Check sheet for the modelled part. Datum: model origin and axes. Units: mm. Face numbers are marked on the shaded views. A direction names the side the tool comes from. Give positions to 0.01 mm unless a question says otherwise; leave off trailing zeros. Loops run counter-clockwise (first coordinate to the right, second up) from the corner with the lowest first, then second, coordinate; pieces in that order, holes last.
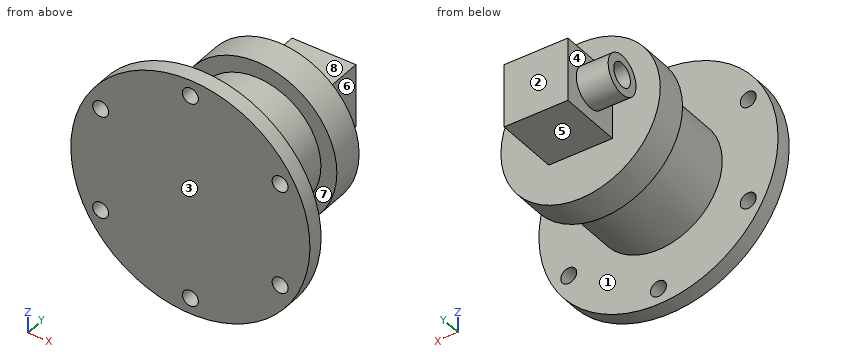
```python
from build123d import *

# Parameters (mm, degrees)
SKETCH1_R           = 75
BOSS_EXTRUDE1_DEPTH = 10
SKETCH2_R           = 5
CUT_EXTRUDE1_DEPTH  = 10
SKETCH3_R           = 40
BOSS_EXTRUDE2_DEPTH = 50
SKETCH4_R           = 50
BOSS_EXTRUDE3_DEPTH = 20
SKETCH5_W           = 40
SKETCH5_H           = 40
BOSS_EXTRUDE4_DEPTH = 40
SKETCH6_R           = 12.5
BOSS_EXTRUDE5_DEPTH = 20
SKETCH9_R           = 7.5
CUT_EXTRUDE2_DEPTH  = 15


with BuildPart() as part:
    # Sketch1 → Boss-Extrude1 (new body)
    with BuildSketch(Plane(origin=(0, 0, 0), x_dir=(1, 0, 0), z_dir=(0, 1, 0))):
        with Locations(Location((0, 0, 0), (0, 0, 270))):
            Circle(SKETCH1_R)
    extrude(amount=BOSS_EXTRUDE1_DEPTH)

    # Sketch2 → Cut-Extrude1 (cut)
    with BuildSketch(Plane(origin=(0, 10, 0), x_dir=(1, 0, 0), z_dir=(0, 1, 0))):
        with Locations(Location((0, 65, 0), (0, 0, 270))):
            Circle(SKETCH2_R)
        with Locations(Location((56.291651246, 32.5, 0), (0, 0, 270))):
            Circle(SKETCH2_R)
        with Locations(Location((56.291651246, -32.5, 0), (0, 0, 270))):
            Circle(SKETCH2_R)
        with Locations(Location((0, -65, 0), (0, 0, 270))):
            Circle(SKETCH2_R)
        with Locations(Location((-56.291651246, -32.5, 0), (0, 0, 270))):
            Circle(SKETCH2_R)
        with Locations(Location((-56.291651246, 32.5, 0), (0, 0, 270))):
            Circle(SKETCH2_R)
    extrude(amount=-CUT_EXTRUDE1_DEPTH, mode=Mode.SUBTRACT)

    # Sketch3 → Boss-Extrude2 (add)
    with BuildSketch(Plane(origin=(0, 10, 0), x_dir=(1, 0, 0), z_dir=(0, 1, 0))):
        with Locations(Location((0, 0, 0), (0, 0, 270))):
            Circle(SKETCH3_R)
    extrude(amount=BOSS_EXTRUDE2_DEPTH)

    # Sketch4 → Boss-Extrude3 (add)
    with BuildSketch(Plane(origin=(0, 60, 0), x_dir=(1, 0, 0), z_dir=(0, 1, 0))):
        with Locations(Location((0, 0, 0), (0, 0, 270))):
            Circle(SKETCH4_R)
    extrude(amount=BOSS_EXTRUDE3_DEPTH)

    # Sketch5 → Boss-Extrude4 (add)
    with BuildSketch(Plane(origin=(0, 80, 0), x_dir=(1, 0, 0), z_dir=(0, 1, 0))):
        Rectangle(SKETCH5_W, SKETCH5_H)
    extrude(amount=BOSS_EXTRUDE4_DEPTH)

    # Sketch6 → Boss-Extrude5 (add)
    with BuildSketch(Plane.ZY.offset(20)):
        with Locations(Location((0, 100, 0), (0, 0, 180))):
            Circle(SKETCH6_R)
    extrude(amount=BOSS_EXTRUDE5_DEPTH)

    # Sketch9 → Cut-Extrude2 (cut)
    with BuildSketch(Plane.ZY.offset(40)):
        with Locations((0, 100)):
            Circle(SKETCH9_R)
    extrude(amount=-CUT_EXTRUDE2_DEPTH, mode=Mode.SUBTRACT)


solid = part.part
```
(1) Section check A-A on z = 32.5. Record the boundary of the cut face in (x, y), plus the area to 3 significant figures.
(2) Section check B-B on z = 65. Record the boundary of the cut face in (x, y).
(3) Access from +Z, -Z, +X, -X, +Y, -Y to the whole of each face (thin tool, end or side, straight path). Record for the marked faces 4, 5, 6, 7 and 8.
(4) Release check for a two-part mould opening along Y. For the marked faces 1, 2 and 3 record: pulls with the +Y half, pulls with the -Y half, needs draft (parallel to the pull), parting line crosses it, or undercut.
(5) Gauge pin test, flat ends, axial feed: pin 1 Ø19.5 at (y, z) = (100, 0) entering from -X; pin 2 Ø6 at (x, y) = (31, 84) entering from -Z; pin 3 Ø5 at (x, z) = (26, 44) entering from +Y; pin 4 Ø8 at (x, y) = (26, 65) entering from +Z. Record the tip position at first contact, or that the pin passes through.
(6) Section check C-C on y = 100. Record the boundary of the cut face in (x, z), plus the area to 4 significant figures.
(7) Material ranges on line 1 (Y direction, x = -33, z = -28.5); line 2 (X direction, y = 3.75, z = 32.5); line 3 (X direction, y = 3, z = -32), recorded low to high.
(8) Section check D-D on x = 59. Record the boundary of the cut face in (y, z).
Computed values:
1. outline: (-67.59, 0) - (-61.29, 0) - (-61.29, 10) - (-67.59, 10) - close; (-51.29, 0) - (51.29, 0) - (51.29, 10) - (23.32, 10) - (23.32, 60) - (38, 60) - (38, 80) - (-38, 80) - (-38, 60) - (-23.32, 60) - (-23.32, 10) - (-51.29, 10) - close; (61.29, 0) - (67.59, 0) - (67.59, 10) - (61.29, 10) - close
1. area: 5,000 mm2
2. outline: (-37.42, 0) - (-5, 0) - (-5, 10) - (-37.42, 10) - close; (5, 0) - (37.42, 0) - (37.42, 10) - (5, 10) - close
3. face 4: -X
3. face 5: -Z, +X, -X, +Y
3. face 6: +Z, -Z, +X, +Y
3. face 7: none
3. face 8: +Z, +X, -X, +Y
4. face 1: undercut
4. face 2: pulls with the +Y half
4. face 3: pulls with the -Y half
5. pin 1: stops at x = -40
5. pin 2: passes through
5. pin 3: stops at y = 80
5. pin 4: stops at z = 44.9
6. outline: (-40, -12.5) - (-20, -12.5) - (-20, -20) - (20, -20) - (20, 20) - (-20, 20) - (-20, 12.5) - (-40, 12.5) - (-40, 7.5) - (-25, 7.5) - (-25, -7.5) - (-40, -7.5) - close
6. area: 1,875 mm2
7. line 1: y = 0 to 10, 60 to 80
7. line 2: x = -67.59 to -61.29, -51.29 to 51.29, 61.29 to 67.59
7. line 3: x = -67.83 to -61.27, -51.32 to 51.32, 61.27 to 67.83
8. outline: (0, -46.3) - (10, -46.3) - (10, -36.7) - (0, -36.7) - close; (0, -28.3) - (10, -28.3) - (10, 28.3) - (0, 28.3) - close; (0, 36.7) - (10, 36.7) - (10, 46.3) - (0, 46.3) - close
